Design review of the part built by this model. Coordinates are the model's own, in mm. A direction names the side the tool comes from. Coordinates: 2 decimals unless noted, no trailing zeros. Write each loop counter-clockwise with the first axis right and the second up, starting at its lowest first coordinate (ties: lowest second). Pieces come first, ordered by that corner, then holes. Notation, with made-up numbers: (9, 17.25) - (24, 17.25) arc R20 cw to (24, 41.25) - close; hole circle Ø9 at (-29, 69.5). An arc over 180 degrees is marked (long way). Answer as a JSON object with one key per item and string values.
Autodesk Inventor part; units mm, degrees
ref_plane "Arbeitsebene2" through (-72, 28.2506, 5) normal (0, 0, -1) x (0, 1, 0)
ref_plane "YZ Plane" through (0, 0, 0) normal (1, 0, 0) x (0, 1, 0)
ref_plane "XZ Plane" through (0, 0, 0) normal (0, 1, 0) x (-1, 0, 0)
ref_plane "Arbeitsebene1" through (0, 0, 0) normal (0, 0, 1) x (1, 0, 0)
sketch "Skizze1" plane through (0, 0, 0) normal (0, 0, 1) x (1, 0, 0)
  line L0 (15, 26.0506) -> (15, 58.2506)
  line L1 (15, 58.2506) -> (-15, 58.2506)
  line L2 (-15, 58.2506) -> (-15, 26.0506)
  line L3 (-15, 26.0506) -> (15, 26.0506)
  circle A0 centre (10, 32.1506) radius 1.25 construction
  circle A1 centre (-10, 32.1506) radius 1.25 construction
  circle A2 centre (-10, 52.1506) radius 1.25 construction
  circle A3 centre (10, 52.1506) radius 1.25 construction
  circle A4 centre (7.5, 38.0506) radius 3.25 construction
  circle A5 centre (7.5, 46.2506) radius 3.25 construction
  circle A6 centre (-7.5, 38.0506) radius 3.25 construction
  circle A7 centre (-7.5, 46.2506) radius 3.25 construction
  line L4 (-65, 27.1506) -> (-65, 57.1506)
  circle A8 centre (10, 32.1506) radius 1.25
  circle A9 centre (-10, 32.1506) radius 1.25
  circle A10 centre (-10, 52.1506) radius 1.25
  circle A11 centre (10, 52.1506) radius 1.25
  line L5 (15, 58.2506) -> (25, 58.2506)
  line L6 (25, 58.2506) -> (25, 26.0506)
  line L7 (25, 26.0506) -> (15, 26.0506)
  line L8 (15, 26.0506) -> (15, 58.2506)
  line L9 (-15, 58.2506) -> (-25, 58.2506)
  line L10 (-25, 58.2506) -> (-25, 26.0506)
  line L11 (-25, 26.0506) -> (-15, 26.0506)
  line L12 (-15, 26.0506) -> (-15, 58.2506)
  line L13 (25, 26.0506) -> (-25, 26.0506)
  line L14 (-25, 26.0506) -> (-25, 22.0506)
  line L15 (-25, 22.0506) -> (25, 22.0506)
  line L16 (25, 22.0506) -> (25, 26.0506)
  line L17 (25, 58.2506) -> (-25, 58.2506)
  line L18 (-25, 58.2506) -> (-25, 62.2506)
  line L19 (-25, 62.2506) -> (25, 62.2506)
  line L20 (25, 62.2506) -> (25, 58.2506)
  point P0 (0, 0)
  dimension "d19" = 10
  dimension "d20" = 10
  dimension "d26" = 4
  dimension "d27" = 4
ref_plane "Arbeitsebene2" through (-72, 28.2506, 5) normal (0, 0, -1) x (0, 1, 0)
extrude "Extrusion1" add sketch "Skizze1" along normal up to surface (5 mm away)
sketch "Skizze2" plane through (-15, 58.2506, 5) normal (0, 0, 1) x (1, 0, 0)
  circle A0 centre (25, -26.1) radius 1.25
  circle A1 centre (5, -26.1) radius 1.25
  circle A2 centre (5, -6.1) radius 1.25
  circle A3 centre (25, -6.1) radius 1.25
  point P0 (15, -58.2506)
hole "Bohrung1" at (10, 32.1506, 5) at (-10, 32.1506, 5) at (-10, 52.1506, 5) at (10, 52.1506, 5) direction (0, 0, -1) diameter 2.8 end through all counterbore diameter 7 counterbore depth 3
sketch "Skizze3" plane through (-15, 58.2506, 5) normal (0, 0, 1) x (1, 0, 0)
  circle A0 centre (14.8208, -23.6) radius 1.7
  circle A1 centre (14.8208, -8.6) radius 1.7
  circle A2 centre (5, -6.1) radius 3.5
  circle A3 centre (25, -26.1) radius 3.5
  circle A4 centre (5, -26.1) radius 3.5
  circle A5 centre (25, -6.1) radius 3.5
  line L0 (-10, 0) -> (-10, -32.2)
  line L1 (-10, -16.1) -> (40, -16.1)
  line L2 (40, -32.2) -> (40, 0)
  circle A6 centre (14.8208, -5.1) radius 1.5853
  circle A7 centre (14.8208, -27.1) radius 2.0333
  point P0 (15, -58.2506)
  dimension "d24" = 11
  dimension "d25" = 11
hole "Bohrung2" at (-0.1792, 31.1506, 5) at (-0.1792, 53.1506, 5) direction (0, 0, -1) diameter 2.8 end through all
pattern_linear "Rechteckige Anordnung1" count 3 spacing 19 along (-1, 0, 0) of "Bohrung2" first direction both ways yes
sketch "Skizze5" plane through (-25, 62.2506, 5) normal (0, 0, 1) x (1, 0, 0)
  line L0 (-41, -5.1) -> (47, -5.1)
  line L1 (-24.541, -42.8) -> (44.8306, -42.8)
  line L2 (16.25, -40.0792) -> (10.75, -40.0792)
  line L3 (0, -40.2) -> (50, -40.2)
  line L4 (50, 0) -> (0, 0)
  line L5 (-41, -35.1) -> (47, -35.1)
  line L6 (50, 0) -> (0, 0)
  line L7 (0, 0) -> (0, -5.1)
  line L8 (0, -5.1) -> (50, -5.1)
  line L9 (50, -5.1) -> (50, 0)
  line L10 (0, -40.2) -> (50, -40.2)
  line L11 (0, 0) -> (0, -40.2)
  line L12 (50, -40.2) -> (0, -40.2)
  line L13 (0, -40.2) -> (0, -35.1)
  line L14 (0, -35.1) -> (50, -35.1)
  line L15 (50, -35.1) -> (50, -40.2)
  point P0 (25, -62.2506)
  point P1 (47, -5.1)
extrude "Extrusion3" add sketch "Skizze5" along normal blind 6 draft -2
sketch "Skizze6" plane through (0, 0, 0) normal (0, 0, -1) x (-1, 0, 0)
  circle A0 centre (19.1792, 31.1506) radius 1.4
  circle A1 centre (19.1792, 53.1506) radius 1.4
  circle A2 centre (-18.8208, 31.1506) radius 1.4
  circle A3 centre (-18.8208, 53.1506) radius 1.4
  circle A4 centre (0.1792, 31.1506) radius 1.4
  circle A5 centre (0.1792, 53.1506) radius 1.4
  circle A6 centre (10, 52.1506) radius 1.4
  circle A7 centre (-10, 32.1506) radius 1.4
  circle A8 centre (10, 32.1506) radius 1.4
  circle A9 centre (-10, 52.1506) radius 1.4
  line L0 (25, 62.2506) -> (25, 22.0506)
  line L1 (-25, 62.2506) -> (25, 62.2506)
  line L2 (-25, 22.0506) -> (-25, 62.2506)
  line L3 (25, 22.0506) -> (-25, 22.0506)
  point P0 (0, 0)
extrude "Extrusion4" add sketch "Skizze6" along normal blind 2
properties part number "20_Cube_Insert_Linear_Stage_NEMA11_china_xymount"
(1) Take a section at B-B, the plane z = 9.5. Write out the cut boundary in (x, y).
Solved:
{"outline": "(-24.84, 22.21) - (24.84, 22.21) - (24.84, 26.99) - (-24.84, 26.99) - close; (-24.84, 57.31) - (24.84, 57.31) - (24.84, 62.09) - (-24.84, 62.09) - close"}
(2) To check wall thickness, follow line 1 (Y direction, x = -19, z = 0); line 2 (Y direction, x = -10, z = 3.3); line 3 (Z direction, x = -8, y = 54). State the ranges of each line that lie inside material, in increasing order. Write a range as from..to.
Solved:
{"line 1": "y = 22.05..29.76, 32.54..51.76, 54.54..62.25", "line 2": "y = 22.05..28.65, 35.65..48.65, 55.65..62.25", "line 3": "z = -2..2"}
(3) For pin 1 (3.5 mm diameter, centred on x = 10.5, y = 33, fed in from +Z); pin 2 (2.5 mm diameter, centred on x = 18.82, y = 53.15, fed in from -Z); pin 3 (5.5 mm diameter, centred on x = -11.5, y = 51.5, fed in from +Z); pin 4 (1.5 mm diameter, centred on x = -17.5, z = 7, fed in from -Y), all flat-tipped, find the tip position at first contact; note any pin that passes through.
Solved:
{"pin 1": "stops at z = 2", "pin 2": "passes through", "pin 3": "stops at z = 5", "pin 4": "stops at y = 22.09"}
(4) The part is to be moulded in two halves that separate along X. For faces 1 (the face through (-8, 32, 2)), 2 (the face through (-25, 42, 2)), 3 (the face through (0, 25, 11)), say which applies: pulls with the +X half, pulls with the -X half, needs draft (parallel to the pull), parting line crosses it, or undercut.
Solved:
{"face 1": "undercut", "face 2": "pulls with the -X half", "face 3": "needs draft"}
(5) Take a section at A-A, the plane x = -10. Write out the cut boundary in (y, z).
Solved:
{"outline": "(22.05, -2) - (30.75, -2) - (30.75, 2) - (28.65, 2) - (28.65, 5) - (27.15, 5) - (26.94, 11) - (22.26, 11) - (22.05, 5) - close; (33.55, -2) - (50.75, -2) - (50.75, 2) - (48.65, 2) - (48.65, 5) - (35.65, 5) - (35.65, 2) - (33.55, 2) - close; (53.55, -2) - (62.25, -2) - (62.25, 5) - (62.04, 11) - (57.36, 11) - (57.15, 5) - (55.65, 5) - (55.65, 2) - (53.55, 2) - close"}
(6) Take a section at C-C, the plane z = -0.75. Give the number of separate pieces and of enclosed holes in the cut face, and give its area (3 significant figures).
Solved:
{"separate pieces": "1", "enclosed holes": "10", "area": "1,950 mm^2"}
(7) Tool access review of faces 4 (the face through (0, 22.051, 2)), 5 (the face through (12, 32, 2)): name each direction out of +Z, -Z, +X, -X, +Y, -Y from which nothing blocks a thin tool from reaching the whole face with its end or side.
Solved:
{"face 4": "+Z, -Z, +X, -X, -Y", "face 5": "+Z"}
(8) Take a section at D-D, the plane x = -2.5. Write out the cut boundary in (y, z).
Solved:
{"outline": "(22.05, -2) - (62.25, -2) - (62.25, 5) - (62.04, 11) - (57.36, 11) - (57.15, 5) - (27.15, 5) - (26.94, 11) - (22.26, 11) - (22.05, 5) - close"}
